CAD build for the part. Positions are in the model's coordinates, mm. A direction names the side the tool comes from. Coordinates: 2 decimals unless noted, no trailing zeros. Loops run counter-clockwise (first coordinate to the right, second up) from the corner with the lowest first, then second, coordinate; pieces in that order, holes last. Notation, with made-up numbers: (-16.5, 16.5) -> (34.5, 16.5) arc R25 cw to (34.5, 33.5) -> close; hole circle Ø11 at (65, 39.5). An arc over 180 degrees is marked (long way). Return JSON: item names as keys, results as strings. Group by question number.
(1) Probe L1, parallel to Y at x = -14.5, z = 3; L2, parallel to X at y = -11, z = 3.25; L3, parallel to Y at x = 1.5, z = 1.75. List the from-to ranges inside material, lowest first.
(2) Tool access for faces 1 (the face through (-5, 1, 0)), 2 (the face through (15, -35, 3)), 3 (the face through (7.765, -43, 3)): list every direction of +Z, -Z, +X, -X, +Y, -Y with a clear straight run to the whole face (end or side of a thin tool).
(3) Saw through at C-C on z = 3.5. Give the number of separate pieces and of enclosed holes in the cut face, then the cut area to 3 significant figures.
(4) Saw through at D-D on x = -5.5. Write the cut outline in (y, z), then the cut area to 3 significant figures.
(5) Saw through at B-B on y = -41. Write the cut outline in (x, z), then the cut area to 3 significant figures.
(6) Saw through at A-A on y = 7.5. Write the cut outline in (x, z).
(7) Mould opens along Y. For faces 4 (the face through (-17, 48, 3)), 5 (the face through (0, -20, 3)), 6 (the face through (14, -35, 3)), 7 (the face through (18, -47, 3)) say: pulls with the +Y half, pulls with the -Y half, needs draft (parallel to the pull), parting line crosses it, or undercut.
(8) Flat gauge pins, fed straight in: pin 1 Ø1 at (x, z) = (0, 3.5) entering from -Y; pin 2 Ø3 at (x, z) = (0, 4.5) entering from -Y; pin 3 Ø3 at (x, z) = (-0.5, 3) entering from -Y. Where does each tip first touch, or does it go through?
```python
from build123d import *

# Parameters (mm, degrees)
F0_W     = 40
F0_H     = 100
F1_DEPTH = 6.4
F2_SIZE  = 5
F4_DEPTH = 6.401
F5_W     = 1
F5_H     = 4
F6_DEPTH = 6.401
F7_W     = 3.5
F7_H     = 12
F8_DEPTH = 6.401


with BuildPart() as f1:
    # F0 (on Top) → F1 (new body)
    with BuildSketch(Plane.XY):
        Rectangle(F0_W, F0_H)
    extrude(amount=F1_DEPTH)

    # F2
    f2_edges = [f1.edges().sort_by_distance(p)[0] for p in [
        (-20, -50, 3.2),
        (20, -50, 3.2),
        (20, 50, 3.2),
        (-20, 50, 3.2),
    ]]
    chamfer(f2_edges, length=F2_SIZE)

    # F3 (on face) → F4 (cut, through all)
    with BuildSketch(Plane.XY.offset(6.4)):
        Polygon((3.882286, -41.724316), (6.724316, -38.882286), (7.764571, -35), (6.724316, -31.117714), (3.882286, -28.275684), (0, -27.235429), (-3.882286, -28.275684), (-6.724316, -31.117714), (-7.764571, -35), (-6.724316, -38.882286), (-3.882286, -41.724316), (0, -42.764571), align=None)
        Polygon((7.764571, -35), (6.724316, -38.882286), (3.882286, -41.724316), (0, -42.764571), (-3.882286, -41.724316), (-6.724316, -38.882286), (-7.764571, -35), (-7.764571, -50), (7.764571, -50), align=None)
    extrude(amount=-F4_DEPTH, mode=Mode.SUBTRACT)

    # F5 (on face) → F6 (cut, through all)
    with BuildSketch(Plane.XY.offset(6.4)):
        with Locations((14.5, -35)):
            Rectangle(F5_W, F5_H)
        with Locations((-14.5, -35)):
            Rectangle(F5_W, F5_H)
    extrude(amount=-F6_DEPTH, mode=Mode.SUBTRACT)

    # F7 (on face) → F8 (cut, through all)
    with BuildSketch(Plane.XY.offset(6.4)):
        with Locations((0, 6)):
            Rectangle(F7_W, F7_H)
        with Locations((0, -14)):
            Rectangle(F7_W, F7_H)
        with Locations((0, 26)):
            Rectangle(F7_W, F7_H)
    extrude(amount=-F8_DEPTH, mode=Mode.SUBTRACT)


solid = f1.part
```
Geometry results:
{
 "1": {"L1": "-50 to -37, -33 to 50", "L2": "-20 to -1.75, 1.75 to 20", "L3": "-27.64 to -20, -8 to 0, 12 to 20, 32 to 50"},
 "2": {"face 1": "-Z, +X, -X, +Y, -Y", "face 2": "+Z, -Z", "face 3": "+Z, -Z, -Y"},
 "3": {"separate pieces": "1", "enclosed holes": "5", "area": "3,490 mm²"},
 "4": {"outline": "(-29.89, 0) -> (50, 0) -> (50, 6.4) -> (-29.89, 6.4) -> close", "area": "511 mm²"},
 "5": {"outline": "(-20, 0) -> (-7.76, 0) -> (-7.76, 6.4) -> (-20, 6.4) -> close; (7.76, 0) -> (20, 0) -> (20, 6.4) -> (7.76, 6.4) -> close", "area": "157 mm²"},
 "6": {"outline": "(-20, 0) -> (-1.75, 0) -> (-1.75, 6.4) -> (-20, 6.4) -> close; (1.75, 0) -> (20, 0) -> (20, 6.4) -> (1.75, 6.4) -> close"},
 "7": {"face 4": "pulls with the +Y half", "face 5": "undercut", "face 6": "undercut", "face 7": "pulls with the -Y half"},
 "8": {"pin 1": "y = -27.37", "pin 2": "y = -27.64", "pin 3": "y = -27.77"}
}
